Verification items for the finished model (mm, model axes). Face numbers are marked on the shaded views. A direction names the side the tool comes from. Give positions to 0.01 mm unless a question says otherwise; leave off trailing zeros. Write each loop counter-clockwise with the first axis right and the second up, starting at its lowest first coordinate (ties: lowest second). Pieces come first, ordered by that corner, then holes. Notation, with made-up numbers: (34.25, -39.75) - (60.25, -39.75) arc R31 cw to (60.25, -5.75) - close; hole circle Ø2 at (-9.75, 18.5). An arc over 180 degrees is marked (long way). Answer as a JSON object with one key per item and string values. Group by question number.
Item 1: Draft check along X on the marked faces 1, 2, 3 and 4. Enter one of: +X half, -X half, draft (parallel to the pull), parting line (faces both ways), or undercut.
Item 2: Sectioned sample at D-D, the plane z = -39.5. Record the boundary of the cut face in (x, y), and give its area (3 significant figures).
Item 3: Sectioned sample at B-B, the plane y = -3. Record the boundary of the cut face in (x, z).
Item 4: Scan lines: line 1 along Y through (x, z) = (17, -32); line 2 along Z through (x, y) = (18.5, 7); line 3 along Z through (x, y) = (3.5, 1). Record each from-to range of solid material in increasing order. Write a range as [from, to].
Item 5: Sectioned sample at C-C, the plane x = 14.5. Record the boundary of the cut face in (y, z), and give its area (3 significant figures).
Item 6: Tool access check on the marked faces 5, 6 and 7. Record the directions out of +Z, -Z, +X, -X, +Y, -Y that give a thin tool (end or side, any length) a straight path to the whole face; none if there is none.
Item 7: Go/stop test with flat-tipped pins: pin 1 (3 mm diameter, centred on x = 2.5, y = 13, fed in from +Z); pin 2 (9.5 mm diameter, centred on y = 12, z = -9, fed in from +X); pin 3 (6.5 mm diameter, centred on x = -1.5, z = -56, fed in from +Y). Record where each tip stops, or that it passes through.
Item 8: Sectioned sample at A-A, the plane y = 1. Count the separate pieces of the cut face and the enclosed holes in it, and give its area (3 significant figures).
```python
from build123d import *

# Parameters (mm, degrees)
EXTRUDE1_DEPTH      = 20.6375
EXTRUDE1_DEPTH_BACK = 20.6375
CUT_EXTRUDE1_REACH  = 27.4
SKETCH4_R           = 7.99973
SKETCH4_R_2         = 4.3688
EXTRUDE2_DEPTH      = 9.144
EXTRUDE3_DEPTH      = 7.925
EXTRUDE3_DEPTH_BACK = 7.925
CUT_EXTRUDE2_DEPTH  = 24.765
LPATTERN2_COUNT     = 3
LPATTERN2_PITCH     = 1.5875
FILLET1_R           = 0.7874
SKETCH11_R          = 3.3145
CUT_EXTRUDE3_DEPTH  = 4.7498


with BuildPart() as part:
    # Sketch1 → Extrude1 (new body, two sides)
    with BuildSketch(Plane(origin=(0, 0, 0), x_dir=(0, 0, -1), z_dir=(1, 0, 0))) as extrude1_sk:
        Polygon((44.45, 25.4), (68.273015024, 19.016642363), (68.273015024, 12.442638617), (70.6374, 11.809103573), (70.6374, 0), (0, 0), (0, 25.4), align=None)
    extrude(amount=EXTRUDE1_DEPTH)
    extrude(extrude1_sk.sketch, amount=-EXTRUDE1_DEPTH_BACK)

    # Cut-Extrude1: up to this plane
    cut_extrude1_end = Plane(origin=(-20.6375, 12.442638617, -68.273015024), z_dir=(0, 0.965925826, -0.258819045))
    # Sketch2 → Cut-Extrude1 (cut, up to the surface)
    with BuildSketch(Plane.XZ, mode=Mode.PRIVATE) as cut_extrude1_sk1:
        with BuildLine():
            Line((20.6375, -70.6374), (12.7, -70.6374))
            ThreePointArc((12.7, -70.6374), (13.832391453, -68.932629596), (15.769776585, -68.273015024))
            Line((15.769776585, -68.273015024), (20.6375, -68.273015024))
            Line((20.6375, -68.273015024), (20.6375, -70.6374))
        make_face()
    cut_extrude1_tool1 = split(extrude(cut_extrude1_sk1.sketch, amount=-CUT_EXTRUDE1_REACH, mode=Mode.PRIVATE), bisect_by=cut_extrude1_end, keep=Keep.BOTH, mode=Mode.PRIVATE)
    add(cut_extrude1_tool1.solids().sort_by_distance((17.033922, 0, -69.518139))[0], mode=Mode.SUBTRACT)
    # Sketch2 → Cut-Extrude1 (cut, up to the surface)
    with BuildSketch(Plane.XZ, mode=Mode.PRIVATE) as cut_extrude1_sk2:
        with BuildLine():
            Line((-20.6375, -68.273015024), (-15.769776585, -68.273015024))
            ThreePointArc((-15.769776585, -68.273015024), (-13.832391453, -68.932629596), (-12.7, -70.6374))
            Line((-12.7, -70.6374), (-20.6375, -70.6374))
            Line((-20.6375, -70.6374), (-20.6375, -68.273015024))
        make_face()
    cut_extrude1_tool2 = split(extrude(cut_extrude1_sk2.sketch, amount=-CUT_EXTRUDE1_REACH, mode=Mode.PRIVATE), bisect_by=cut_extrude1_end, keep=Keep.BOTH, mode=Mode.PRIVATE)
    add(cut_extrude1_tool2.solids().sort_by_distance((-17.033922, 0, -69.518139))[0], mode=Mode.SUBTRACT)

    # Sketch3 → Cut-Revolve1 (revolve, cut)
    with BuildSketch(Plane(origin=(0, 0, 0), x_dir=(0, 0, -1), z_dir=(1, 0, 0)), mode=Mode.PRIVATE) as cut_revolve1_sk:
        Polygon((49.5937, 24.021749739), (49.5937, 17.232918978), (51.8412, 17.232918978), (51.8412, 3.175), (48.3616, 3.175), (48.3616, 0), (56.3372, 0), (56.3372, 24.021749739), align=None)
    revolve(cut_revolve1_sk.sketch.rotate(Axis((0, -4.910727806, -56.3372), (0, 1, 0)), 180), axis=Axis((0, -4.910727806, -56.3372), (0, 1, 0)), mode=Mode.SUBTRACT)  # turned: the seam where the file's is

    # Sketch4 → Extrude2 (add)
    with BuildSketch(Plane.XZ.offset(-3.175)):
        with Locations(Location((0, -56.3372, 0), (0, 0, 270))):  # turned: the seam where the file's is
            Circle(SKETCH4_R)
        with Locations(Location((0, -56.3372, 0), (0, 0, 270))):  # turned: the seam where the file's is
            Circle(SKETCH4_R_2, mode=Mode.SUBTRACT)
    extrude(amount=EXTRUDE2_DEPTH)

    # Sketch6 → Extrude3 (add, two sides)
    with BuildSketch(Plane(origin=(0, 0, 0), x_dir=(0, 0, -1), z_dir=(1, 0, 0))) as extrude3_sk:
        Polygon((70.6374, 2.789570434), (75.4126, 1.51005945), (75.4126, 8.12340369), (70.6374, 9.402914674), align=None)
    extrude(amount=EXTRUDE3_DEPTH)
    extrude(extrude3_sk.sketch, amount=-EXTRUDE3_DEPTH_BACK)

    # Sketch7 → Cut-Extrude2 (cut, symmetric)
    with BuildSketch(Plane(origin=(0, 0, 0), x_dir=(0, 0, -1), z_dir=(1, 0, 0))):
        Polygon((75.4126, 3.49443445), (75.4126, 2.70068445), (74.61885, 2.913369121), (74.61885, 3.281749778), align=None)
    cut_extrude2 = extrude(amount=CUT_EXTRUDE2_DEPTH, both=True, mode=Mode.SUBTRACT)

    # LPattern2: Cut-Extrude2 ×3
    with Locations(*[(0, i * LPATTERN2_PITCH, 0) for i in range(1, LPATTERN2_COUNT)]):
        add(cut_extrude2, mode=Mode.SUBTRACT)

    # Fillet1
    fillet1_edges = [part.edges().sort_by_distance(p)[0] for p in [
        (0, 8.12340369, -75.4126),
        (0, 1.51005945, -75.4126),
    ]]
    fillet(fillet1_edges, radius=FILLET1_R)

    # Sketch11 → Cut-Extrude3 (cut)
    with BuildSketch(Plane.XZ):
        with Locations(Location((0, -8.7122, 0), (0, 0, 270))):  # turned: the seam where the file's is
            Circle(SKETCH11_R)
    extrude(amount=-CUT_EXTRUDE3_DEPTH, mode=Mode.SUBTRACT)

    # Sketch12 → Cut-Revolve2 (revolve, cut)
    with BuildSketch(Plane(origin=(0, 0, 0), x_dir=(0, 0, -1), z_dir=(1, 0, 0)), mode=Mode.PRIVATE) as cut_revolve2_sk:
        Polygon((0, 21.7424), (2.54, 21.7424), (2.54, 18.4404), (2.55, 18.4404), (3.0835, 17.9069), (13.106, 17.9069), (13.106, 13.4874), (0, 13.4874), align=None)
    revolve(cut_revolve2_sk.sketch.rotate(Axis((0, 13.4874, 3.668396013), (0, 0, -1)), 180), axis=Axis((0, 13.4874, 3.668396013), (0, 0, -1)), mode=Mode.SUBTRACT)  # turned: the seam where the file's is

    # Sketch13 → Cut-Revolve3 (revolve, cut)
    with BuildSketch(Plane.XY.offset(-11.1252), mode=Mode.PRIVATE) as cut_revolve3_sk:
        Polygon((20.6375, 21.7424), (20.3835, 21.7424), (20.3835, 18.4404), (20.3735, 18.4404), (19.84, 17.9069), (9.8175, 17.9069), (9.8175, 13.4874), (20.6375, 13.4874), align=None)
        Polygon((-20.6375, 13.4874), (-20.6375, 21.7424), (-20.3835, 21.7424), (-20.3835, 18.4404), (-20.3735, 18.4404), (-19.84, 17.9069), (-9.8175, 17.9069), (-9.8175, 13.4874), align=None)
    revolve(cut_revolve3_sk.sketch.rotate(Axis((0, 13.4874, -11.1252), (1, 0, 0)), 90), axis=Axis((0, 13.4874, -11.1252), (1, 0, 0)), mode=Mode.SUBTRACT)  # turned: the seam where the file's is


solid = part.part
```
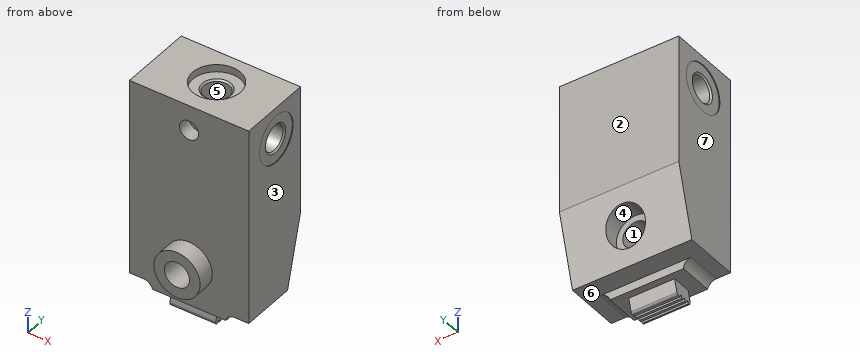
Geometry check:
{
 "1": {"face 1": "undercut", "face 2": "draft", "face 3": "+X half", "face 4": "undercut"},
 "2": {"outline": "(-20.64, 0) - (20.64, 0) - (20.64, 25.4) - (-20.64, 25.4) - close", "area": "1,050 mm^2"},
 "3": {"outline": "circle Ø16 at (0, -56.34); hole circle Ø8.74 at (0, -56.34)"},
 "4": {"line 1": "[0, 25.4]", "line 2": "[-68.27, 0]", "line 3": "[-70.64, -58.95], [-53.72, 0]"},
 "5": {"outline": "(0, -68.54) - (12.37, -68.54) - (12.44, -68.27) - (19.02, -68.27) - (25.4, -44.45) - (25.4, 0) - (0, 0) - close; hole circle Ø8.84 at (13.49, -11.13)", "area": "1,600 mm^2"},
 "6": {"face 5": "+Z", "face 6": "-Z, +Y", "face 7": "+Z, -Z, -X, +Y, -Y"},
 "7": {"pin 1": "z = -13.11", "pin 2": "x = 20.38", "pin 3": "y = 17.23"},
 "8": {"separate pieces": "1", "enclosed holes": "2", "area": "2,790 mm^2"}
}
